For this review, take the finished solid that the model builds, in its own axes (mm). Coordinates: 2 decimals unless noted, no trailing zeros. Order: outer loops, then holes, each group sorted by start corner. A loop starts at its lowest first (then second) coordinate and runs counter-clockwise, first axis right, second up. Notation, with made-up numbers: (41.25, -36.5) -> (90.25, -36.5) arc R29 ccw to (90.25, -10.5) -> close; hole circle Ø4 at (17.25, 45). An arc over 180 degrees is marked (long way). Return JSON: item names as keys, results as strings. Group by question number.
Item 1: Take a section at B-B (z = 30). Write out the cut boundary in (x, y), then the cut area to 3 significant figures.
Item 2: For line 1 along X through (y, z) = (10, 41.5); line 2 along X through (y, z) = (1, 19); line 3 along Z through (x, y) = (-49, -4.5), list the stretches that pass through material, from the lowest coordinate up.
Item 3: Insertion check: pin 1 (1.5 mm diameter, centred on x = 26.5, z = 54.5, fed in from -Y); pin 2 (1.5 mm diameter, centred on y = 13.5, z = 8.5, fed in from +X); pin 3 (3 mm diameter, centred on y = -12.5, z = 34, fed in from +X); pin 4 (1 mm diameter, centred on x = 28.5, y = -20, fed in from +Z). Each pin has a flat end and moves straight along its axis. Give the tip position at first contact, or say it passes through.
Item 4: Take a section at A-A (y = 12). Write out the cut boundary in (x, z), then the cut area to 3 significant figures.
```python
from build123d import *

# Parameters (mm, degrees)
F0_W     = 38.1
F0_H     = 63.5
F1_DEPTH = 25.4
F3_DEPTH = 50.8


# Not quite as in the source:
# - a pattern or mirror of a feature is missing from the dataset's text; its kind, count and spacing are read off the source's solid


with BuildPart() as f1:
    # F0 (on Front) → F1 (new body, symmetric)
    with BuildSketch(Plane.XZ):
        with Locations((0, 31.75)):
            Rectangle(F0_W, F0_H)
    extrude(amount=F1_DEPTH, both=True)

    # F2 (on face) → F3 (join, through all)
    with BuildSketch(Plane.XZ.offset(25.4)):
        Polygon((-19.05, 0), (-19.05, 63.5), (-55.7117420935, 0), align=None)
    f3 = extrude(amount=-F3_DEPTH)

    # F3_copies: F3 across plane
    add(f3.mirror(Plane(origin=(0, 0, 0), x_dir=(0, 0, 1), z_dir=(1, 0, 0))))


solid = f1.part
```
Findings below:
{
 "1": {"outline": "(-38.39, -25.4) -> (38.39, -25.4) -> (38.39, 25.4) -> (-38.39, 25.4) -> close", "area": "3,900 mm2"},
 "2": {"line 1": "x = -31.75 to 31.75", "line 2": "x = -44.74 to 44.74", "line 3": "z = 0 to 11.63"},
 "3": {"pin 1": "passes through", "pin 2": "stops at x = 51.24", "pin 3": "stops at x = 36.95", "pin 4": "stops at z = 48"},
 "4": {"outline": "(-55.71, 0) -> (55.71, 0) -> (19.05, 63.5) -> (-19.05, 63.5) -> close", "area": "4,750 mm2"}
}
